from build123d import *

# Parameters (mm, degrees)
SKETCH_1_R             = 6.25
SM_BASE_FLANGE_1_DEPTH = 6


# Sheet-metal steps are written as plain solids
with BuildPart() as part:
    # Sketch 1 → Базовая кромка1 (new body)
    with BuildSketch(Plane.XY):
        with BuildLine():
            Line((-12, -15), (12, -15))
            ThreePointArc((12, -15), (14.121320344, -14.121320344), (15, -12))
            Line((15, -12), (15, 12))
            ThreePointArc((15, 12), (14.121320344, 14.121320344), (12, 15))
            Line((12, 15), (-12, 15))
            ThreePointArc((-12, 15), (8.423008458, 72.651269477), (52.225050565, 115.337909706))
            ThreePointArc((52.225050565, 115.337909706), (65.873295621, 116.29514987), (74.621175956, 105.775383166))
            Line((74.621175956, 105.775383166), (107.314124719, -40.33280529))
            ThreePointArc((107.314124719, -40.33280529), (105.342791215, -51.642791703), (95.951479838, -58.246216503))
            ThreePointArc((95.951479838, -58.246216503), (59.983147908, -62.22117964), (24.014815979, -58.246216503))
            ThreePointArc((24.014815979, -58.246216503), (19.049536185, -56.141802219), (15.149410164, -52.417345221))
            Line((15.149410164, -52.417345221), (-12, -15))
        make_face()
        with Locations((59.983147908, 102.5)):
            Circle(SKETCH_1_R, mode=Mode.SUBTRACT)
        with Locations((27.290199146, -43.608188456)):
            Circle(SKETCH_1_R, mode=Mode.SUBTRACT)
        with Locations((43.533377705, -46.421825098)):
            Circle(SKETCH_1_R, mode=Mode.SUBTRACT)
        with Locations((59.983147908, -47.5)):
            Circle(SKETCH_1_R, mode=Mode.SUBTRACT)
        with Locations((76.432918112, -46.421825098)):
            Circle(SKETCH_1_R, mode=Mode.SUBTRACT)
        with Locations((92.676096671, -43.608188456)):
            Circle(SKETCH_1_R, mode=Mode.SUBTRACT)
    extrude(amount=SM_BASE_FLANGE_1_DEPTH)


solid = part.part
Geometry: final body of the model. Coordinates: model frame, mm. A direction names the side the tool comes from. Round coordinates to 2 decimals unless told otherwise and drop trailing zeros. Loops run counter-clockwise (first coordinate to the right, second up) from the corner with the lowest first, then second, coordinate; pieces in that order, holes last. Notation, with made-up numbers: M 16.25,-3.75 L 57.25,-3.75 A26 cw 57.25,32.25 Z; hole C 24,28 d5. An arc over 180 degrees is marked long. One line per question, with ' | ' between items.
(1) Cut plane D-D on y = 53. Return the cut outline in (x, z).
Check result:
outline: M -1.98,0 L 86.43,0 L 86.43,6 L -1.98,6 Z
(2) Pull-direction query (X, two-part tool) for faces 3 (the cylindrical face through (105.43, -51.5, 2.96)), 4 (the cylindrical face through (65.69, 116.37, 2.96)), 5 (the cylindrical face through (25.9, -49.7, 3)); classes: +X half, -X half, draft (parallel to the pull), parting line (faces both ways), or undercut.
Check result:
face 3: +X half | face 4: parting line | face 5: undercut
(3) Cut plane C-C on y = -1. Return the cut outline in (x, z).
Check result:
outline: M 15,0 L 98.51,0 L 98.51,6 L 15,6 Z
(4) Access query for faces 1 (the flat face through (1.765, -33.971, 2.958)), 2 (the flat face through (0, 15, 3)). Directions: +Z, -Z, +X, -X, +Y, -Y. A direction counts if a zero-diameter tool reaches every point of the face in a straight line with its end or side. Return the directions, or none.
Check result:
face 1: +Z, -Z, -X, -Y | face 2: +Z, -Z, -X
(5) Material intervals for line 1 along X through (y, z) = (-44.5, 3.8); line 2 along Y through (x, z) = (63.5, 3.6); line 3 along Y through (x, z) = (48.5, 0.5), sorted ascending. Write a range as from..to.
Check result:
line 1: x = 9.4..21.1, 33.48..37.59, 49.48..54.5, 65.47..70.49, 82.38..86.49, 98.86..107.65 | line 2: y = -62.18..-52.67, -42.33..97.33, 107.67..117.08 | line 3: y = -61.82..-50.22, -42.63..113
(6) Cut plane B-B on z = 1. Return the cut outline in (x, y).
Check result:
outline: M -12,-15 L 15.15,-52.42 A15 ccw 24.01,-58.25 A164.72 ccw 95.95,-58.25 A15 ccw 107.31,-40.33 L 74.62,105.78 A15 ccw 52.23,115.34 A134.76 ccw -12,15 L 12,15 A3 cw 15,12 L 15,-12 A3 cw 12,-15 Z; hole C 27.29,-43.61 d12.5; hole C 43.53,-46.42 d12.5; hole C 59.98,-47.5 d12.5; hole C 59.98,102.5 d12.5; hole C 76.43,-46.42 d12.5; hole C 92.68,-43.61 d12.5
(7) Cut plane A-A on y = 102.5. Return the cut outline in (x, z), plus the area to 3 significant figures.
Check result:
outline: M 34.43,0 L 53.73,0 L 53.73,6 L 34.43,6 Z; M 66.23,0 L 75.35,0 L 75.35,6 L 66.23,6 Z | area: 171 mm2
(8) Contact query for flat-ended pins moving along their axis: P1, Ø1.8, axis at x = 6, z = 3, coming from the -Y side; P2, Ø1.5, axis at y = 20, z = 5, coming from the -X side. Output: stop coordinate, or through.
Check result:
P1: stops at y = -41.05 | P2: stops at x = -11.46
